Geometry: final body of the model. Coordinates: model frame, mm. A direction names the side the tool comes from. Round coordinates to 2 decimals unless told otherwise and drop trailing zeros. Loops run counter-clockwise (first coordinate to the right, second up) from the corner with the lowest first, then second, coordinate; pieces in that order, holes last. Notation, with made-up numbers: (15, 70) -> (66, 70) arc R12 cw to (66, 87) -> close; hole circle Ø2 at (20, 13.5). An arc over 180 degrees is marked (long way). Answer in a Markdown table with one row per item.
```python
from build123d import *

# Parameters (mm, degrees)
F0_W     = 40
F0_H     = 40
F1_DEPTH = 40
F2_R     = 12.32
F3_DEPTH = 20


with BuildPart() as f1:
    # F0 (on Top) → F1 (new body)
    with BuildSketch(Plane.XY):
        Rectangle(F0_W, F0_H)
    extrude(amount=F1_DEPTH)

    # F2 (on Front) → F3 (cut)
    with BuildSketch(Plane.XZ):
        with Locations((0, 20.027552)):
            Circle(F2_R)
    extrude(amount=-F3_DEPTH, mode=Mode.SUBTRACT)


solid = f1.part
```
Item 1: Section query B-B, the plane z = 10. Output: boundary loops of the cut face in (x, y), and give its area (3 significant figures).
Ans:
| item | result |
|---|---|
| outline | (-20, -20) -> (20, -20) -> (20, 20) -> (7.16, 20) -> (7.16, 0) -> (-7.16, 0) -> (-7.16, 20) -> (-20, 20) -> close |
| area | 1,310 mm2 |
Item 2: Section query C-C, the plane y = 5. Output: boundary loops of the cut face in (x, z).
Ans:
| item | result |
|---|---|
| outline | (-20, 0) -> (20, 0) -> (20, 40) -> (-20, 40) -> close; hole circle Ø24.64 at (0, 20.03) |
Item 3: Mould query, pull axis X, two halves, no side actions, for faces 1 (the cylindrical face through (6.62, 9.86, 30.42)), 2 (the flat face through (0, -20, 20)), 3 (the flat face through (-20, 0, 20)). Classes: released by +X, released by -X, zero draft, split by the parting line, or undercut.
Ans:
| item | result |
|---|---|
| face 1 | undercut |
| face 2 | zero draft |
| face 3 | released by -X |
Item 4: Section query A-A, the plane x = 0. Output: boundary loops of the cut face in (y, z).
Ans:
| item | result |
|---|---|
| outline | (-20, 0) -> (20, 0) -> (20, 7.71) -> (0, 7.71) -> (0, 32.35) -> (20, 32.35) -> (20, 40) -> (-20, 40) -> close |
Item 5: Ray query, L1, parallel to Z at x = 0.5, y = 14; L2, parallel to X at y = 9.5, z = 20; L3, parallel to Y at x = -1.5, z = 15. Return the intervals inside material, ascending.
Ans:
| item | result |
|---|---|
| L1 | 0 to 7.72, 32.34 to 40 |
| L2 | -20 to -12.32, 12.32 to 20 |
| L3 | -20 to 0 |
Item 6: First-contact query: P1, Ø4, axis at x = 4.5, z = 23, coming from the +Y side; P2, Ø4, axis at x = 5.5, y = -4, coming from the -Z side. Flat tips, straight axial feed; report the tip coordinate or a pass-through.
Ans:
| item | result |
|---|---|
| P1 | y = 0 |
| P2 | z = 0 |
Item 7: Set-up query: faces 4 (the flat face through (-9, 20, 11)), 5 (the flat face through (0, 0, 20)). Return all of +Z, -Z, +X, -X, +Y, -Y with unobstructed straight access to the full face (end or side cutting, diameter ignored); none if empty.
Ans:
| item | result |
|---|---|
| face 4 | +Z, -Z, +X, -X, +Y |
| face 5 | +Y |
